Verification items for the finished model (mm, model axes). A direction names the side the tool comes from. Give positions to 0.01 mm unless a question says otherwise; leave off trailing zeros. Loops run counter-clockwise (first coordinate to the right, second up) from the corner with the lowest first, then second, coordinate; pieces in that order, holes last. Notation, with made-up numbers: (81, 89) - (87, 89) arc R35 ccw to (87, 122) - close; hole circle Ø4 at (-8, 12.25). An arc over 180 degrees is marked (long way). Use one line per item in the form item = value.
```python
from build123d import *

# Parameters (mm, degrees)
SKETCH1_W               = 58.8
SKETCH1_H               = 8
BOSS_EXTRUDE1_DEPTH     = 25
BOSS_EXTRUDE1_2_DEPTH   = 25
SKETCH1_3_W             = 58.8
SKETCH1_3_H             = 33.8
SKETCH1_3_W_2           = 58.5
SKETCH1_3_H_2           = 33.5
BOSS_EXTRUDE2_DEPTH     = 5
SKETCH2_R               = 1.375
CUT_EXTRUDE1_DEPTH      = 5
CUT_EXTRUDE2_DEPTH      = 74
CUT_EXTRUDE2_DEPTH_BACK = 20
SKETCH3_R               = 1.375
SKETCH4_W               = 15
SKETCH4_H               = 15
CUT_EXTRUDE3_DEPTH      = 75
SKETCH5_W               = 49.8
SKETCH5_H               = 25
BOSS_EXTRUDE3_DEPTH     = 8
SKETCH6_R               = 1.375
CUT_EXTRUDE4_DEPTH      = 16
BOSS_EXTRUDE4_START     = 5
SKETCH7_W               = 66.8
SKETCH7_H               = 49.8
SKETCH7_R               = 1.375
BOSS_EXTRUDE4_DEPTH     = 5
SKETCH8_W               = 126.8
SKETCH8_H               = 109.8
SKETCH8_W_2             = 66.8
SKETCH8_H_2             = 49.8
BOSS_EXTRUDE5_DEPTH     = 10
BOSS_EXTRUDE6_DEPTH     = 15
SKETCH11_R              = 1.375
CUT_EXTRUDE5_DEPTH      = 55
SKETCH12_R              = 1.625
CUT_EXTRUDE6_DEPTH      = 55
SKETCH13_R              = 3
CUT_EXTRUDE7_DEPTH      = 5
CUT_EXTRUDE8_START      = -5
SKETCH14_R              = 3
CUT_EXTRUDE8_DEPTH      = 5
SKETCH15_R              = 3
CUT_EXTRUDE9_DEPTH      = 7
SKETCH16_R              = 4
CUT_EXTRUDE10_DEPTH     = 5
SKETCH17_R              = 3
CUT_EXTRUDE11_DEPTH     = 5
BODY_MOVE_COPY1_ANGLE   = 120


with BuildPart() as part:
    # Sketch1 → Boss-Extrude1 (new body)
    with BuildSketch(Plane(origin=(0, 0, 0), x_dir=(1, 0, 0), z_dir=(0, 1, 0))):
        with Locations((0, 20.9)):
            Rectangle(SKETCH1_W, SKETCH1_H)
    extrude(amount=BOSS_EXTRUDE1_DEPTH)



with BuildPart() as body_2:
    # Sketch1 → Boss-Extrude1 2 (new body)
    with BuildSketch(Plane(origin=(0, 0, 0), x_dir=(1, 0, 0), z_dir=(0, 1, 0))):
        with Locations((0, -20.9)):
            Rectangle(SKETCH1_W, SKETCH1_H)
    extrude(amount=BOSS_EXTRUDE1_2_DEPTH)


with BuildPart() as part_1:
    add(part.part)

    add(body_2.part)  # Boss-Extrude2 merges body 2
    # Sketch1_3 → Boss-Extrude2 (add)
    # profile 1 of 2: a face of its own
    with BuildSketch(Plane(origin=(0, 0, 0), x_dir=(1, 0, 0), z_dir=(0, 1, 0))):
        Rectangle(SKETCH1_3_W, SKETCH1_3_H)
        Rectangle(SKETCH1_3_W_2, SKETCH1_3_H_2, mode=Mode.SUBTRACT)
    # profile 2 of 2: a face of its own
    with BuildSketch(Plane(origin=(0, 0, 0), x_dir=(1, 0, 0), z_dir=(0, 1, 0))):
        Rectangle(SKETCH1_3_W_2, SKETCH1_3_H_2)
    extrude(amount=BOSS_EXTRUDE2_DEPTH)

    # Sketch2 → Cut-Extrude1 (cut)
    with BuildSketch(Plane.XZ):
        with Locations(Location((-26.05, 13.5, 0), (0, 0, 270))):
            Circle(SKETCH2_R)
        with Locations(Location((-26.05, -13.5, 0), (0, 0, 270))):
            Circle(SKETCH2_R)
        with Locations(Location((25.95, -13.5, 0), (0, 0, 270))):
            Circle(SKETCH2_R)
        with Locations(Location((25.95, 13.5, 0), (0, 0, 270))):
            Circle(SKETCH2_R)
    extrude(amount=-CUT_EXTRUDE1_DEPTH, mode=Mode.SUBTRACT)

    # Sketch3 → Cut-Extrude2 (cut, two sides: drawn at the far end of the back side and taken through both)
    with BuildSketch(Plane(origin=(0, 0, 16.9), x_dir=(-1, 0, 0), z_dir=(0, 0, -1)).offset(-CUT_EXTRUDE2_DEPTH_BACK)):
        with Locations(Location((-22.45, 19, 0), (0, 0, 180))):
            Circle(SKETCH3_R)
        with Locations(Location((9.55, 19, 0), (0, 0, 180))):
            Circle(SKETCH3_R)
    extrude(amount=CUT_EXTRUDE2_DEPTH + CUT_EXTRUDE2_DEPTH_BACK, mode=Mode.SUBTRACT)

    # Sketch4 → Cut-Extrude3 (cut)
    with BuildSketch(Plane(origin=(0, 0, -24.9), x_dir=(-1, 0, 0), z_dir=(0, 0, -1))):
        with Locations((-1.9, 12.5)):
            Rectangle(SKETCH4_W, SKETCH4_H)
    extrude(amount=-CUT_EXTRUDE3_DEPTH, mode=Mode.SUBTRACT)

    # Sketch5 → Boss-Extrude3 (add)
    with BuildSketch(Plane(origin=(29.4, 0, 0), x_dir=(0, 0, -1), z_dir=(1, 0, 0))):
        with Locations((0, 12.5)):
            Rectangle(SKETCH5_W, SKETCH5_H)
    extrude(amount=BOSS_EXTRUDE3_DEPTH)

    # Sketch6 → Cut-Extrude4 (cut)
    with BuildSketch(Plane(origin=(37.4, 0, 0), x_dir=(0, 0, -1), z_dir=(1, 0, 0))):
        with Locations((-10, 19)):
            Circle(SKETCH6_R)
        with Locations((10, 19)):
            Circle(SKETCH6_R)
    extrude(amount=-CUT_EXTRUDE4_DEPTH, mode=Mode.SUBTRACT)

    # Sketch7 → Boss-Extrude4 (add)
    with BuildSketch(Plane.XZ.offset(BOSS_EXTRUDE4_START)):
        with Locations((4, 0)):
            Rectangle(SKETCH7_W, SKETCH7_H)
        with Locations(Location((-26.05, 13.5, 0), (0, 0, 270))):
            Circle(SKETCH7_R, mode=Mode.SUBTRACT)
        with Locations(Location((25.95, 13.5, 0), (0, 0, 270))):
            Circle(SKETCH7_R, mode=Mode.SUBTRACT)
        with Locations(Location((25.95, -13.5, 0), (0, 0, 270))):
            Circle(SKETCH7_R, mode=Mode.SUBTRACT)
        with Locations(Location((-26.05, -13.5, 0), (0, 0, 270))):
            Circle(SKETCH7_R, mode=Mode.SUBTRACT)
    extrude(amount=-BOSS_EXTRUDE4_DEPTH)

    # Sketch8 → Boss-Extrude5 (add)
    with BuildSketch(Plane.XZ.offset(5)):
        with Locations((4, 0)):
            Rectangle(SKETCH8_W, SKETCH8_H)
        with Locations((4, 0)):
            Rectangle(SKETCH8_W_2, SKETCH8_H_2, mode=Mode.SUBTRACT)
    extrude(amount=-BOSS_EXTRUDE5_DEPTH)

    # Sketch9 → Boss-Extrude6 (add)
    with BuildSketch(Plane(origin=(0, 25, 0), x_dir=(1, 0, 0), z_dir=(0, 1, 0))):
        Polygon((37.4, -24.9), (37.4, 24.9), (9.4, 24.9), (9.4, 16.9), (29.4, 16.9), (29.4, -16.9), (9.4, -16.9), (9.4, -24.9), align=None)
    extrude(amount=BOSS_EXTRUDE6_DEPTH)

    # Sketch11 → Cut-Extrude5 (cut)
    with BuildSketch(Plane.XY.offset(24.9)):
        with Locations((22.45, 35)):
            Circle(SKETCH11_R)
    extrude(amount=-CUT_EXTRUDE5_DEPTH, mode=Mode.SUBTRACT)

    # Sketch12 → Cut-Extrude6 (cut)
    with BuildSketch(Plane(origin=(0, 5, 0), x_dir=(1, 0, 0), z_dir=(0, 1, 0))):
        with Locations(Location((-44.4, 39.9, 0), (0, 0, 270))):
            Circle(SKETCH12_R)
        with Locations(Location((52.4, 39.9, 0), (0, 0, 270))):
            Circle(SKETCH12_R)
        with Locations(Location((52.4, -39.9, 0), (0, 0, 270))):
            Circle(SKETCH12_R)
        with Locations(Location((-44.4, -39.9, 0), (0, 0, 270))):
            Circle(SKETCH12_R)
    extrude(amount=-CUT_EXTRUDE6_DEPTH, mode=Mode.SUBTRACT)

    # Sketch13 → Cut-Extrude7 (cut)
    with BuildSketch(Plane.XY.offset(24.9)):
        with Locations((-9.55, 19)):
            Circle(SKETCH13_R)
        with Locations((22.45, 35)):
            Circle(SKETCH13_R)
        with Locations((22.45, 19)):
            Circle(SKETCH13_R)
    extrude(amount=-CUT_EXTRUDE7_DEPTH, mode=Mode.SUBTRACT)

    # Sketch14 → Cut-Extrude8 (cut)
    with BuildSketch(Plane(origin=(0, 0, -24.9), x_dir=(-1, 0, 0), z_dir=(0, 0, -1)).offset(CUT_EXTRUDE8_START)):
        with Locations(Location((-22.45, 35, 0), (0, 0, 180))):
            Circle(SKETCH14_R)
        with Locations(Location((-22.45, 19, 0), (0, 0, 180))):
            Circle(SKETCH14_R)
        with Locations(Location((9.55, 19, 0), (0, 0, 180))):
            Circle(SKETCH14_R)
    extrude(amount=CUT_EXTRUDE8_DEPTH, mode=Mode.SUBTRACT)

    # Sketch15 → Cut-Extrude9 (cut)
    with BuildSketch(Plane.XZ.offset(5)):
        with Locations(Location((-26.05, 13.5, 0), (0, 0, 270))):
            Circle(SKETCH15_R)
        with Locations(Location((25.95, 13.5, 0), (0, 0, 270))):
            Circle(SKETCH15_R)
        with Locations(Location((25.95, -13.5, 0), (0, 0, 270))):
            Circle(SKETCH15_R)
        with Locations(Location((-26.05, -13.5, 0), (0, 0, 270))):
            Circle(SKETCH15_R)
    extrude(amount=-CUT_EXTRUDE9_DEPTH, mode=Mode.SUBTRACT)

    # Sketch16 → Cut-Extrude10 (cut)
    with BuildSketch(Plane(origin=(0, 5, 0), x_dir=(1, 0, 0), z_dir=(0, 1, 0))):
        with Locations(Location((-44.4, 39.9, 0), (0, 0, 270))):
            Circle(SKETCH16_R)
        with Locations(Location((52.4, 39.9, 0), (0, 0, 270))):
            Circle(SKETCH16_R)
        with Locations(Location((52.4, -39.9, 0), (0, 0, 270))):
            Circle(SKETCH16_R)
        with Locations(Location((-44.4, -39.9, 0), (0, 0, 270))):
            Circle(SKETCH16_R)
    extrude(amount=-CUT_EXTRUDE10_DEPTH, mode=Mode.SUBTRACT)

    # Sketch17 → Cut-Extrude11 (cut)
    with BuildSketch(Plane(origin=(37.4, 0, 0), x_dir=(0, 0, -1), z_dir=(1, 0, 0))):
        with Locations((-10, 19)):
            Circle(SKETCH17_R)
        with Locations((10, 19)):
            Circle(SKETCH17_R)
    extrude(amount=-CUT_EXTRUDE11_DEPTH, mode=Mode.SUBTRACT)


with BuildPart() as part_2:
    # Body-Move_Copy1: moved
    add(part_1.part.moved(Location((0, 0, 0))).rotate(Axis((8.5, 13, -4.5), (0.5773502691896252, -0.5773502691896272, -0.5773502691896252)), BODY_MOVE_COPY1_ANGLE))


solid = part_2.part
```
1. Section check D-D, the plane x = 9. Record the cut outline in (y, z), then the cut area to 3 significant figures.
Result set:
outline = (-45.9, -22.5) - (80.9, -22.5) - (80.9, -12.5) - (-7.9, -12.5) - (-7.9, 22.5) - (-15.9, 22.5) - (-15.9, -12.5) - (-45.9, -12.5) - close
area = 1,550 mm²
2. Section check C-C, the plane y = 65.9. Record the cut outline in (x, z) (3 decimals).
Result set:
outline = (-50.9, -22.5) - (-37.525, -22.5) - (-37.525, -17.5) - (-39.9, -17.5) - (-39.9, -12.5) - (-50.9, -12.5) - close; (-34.275, -22.5) - (42.275, -22.5) - (42.275, -17.5) - (39.9, -17.5) - (39.9, -12.5) - (-31.9, -12.5) - (-31.9, -17.5) - (-34.275, -17.5) - close; (45.525, -22.5) - (58.9, -22.5) - (58.9, -12.5) - (47.9, -12.5) - (47.9, -17.5) - (45.525, -17.5) - close
3. Scan lines: probe 1 along X at (y, z) = (-4.45, -20); probe 2 along Y at (x, z) = (17.5, -18); probe 3 along X at (y, z) = (9.5, 11.5). Record each from-to range of solid material in increasing order.
Result set:
probe_1 = -50.9 to -12.5, -6.5 to 14.5, 20.5 to 58.9
probe_2 = -45.9 to -7.45, -1.45 to 44.55, 50.55 to 80.9
probe_3 = -20.9 to -12.9, 20.9 to 28.9
4. Depth check by flat-ended pin: pin 1 Ø9.5 at (y, z) = (-0.95, 17.5) entering from -X; pin 2 Ø5 at (x, y) = (43.9, -30.9) entering from +Z; pin 3 Ø9.5 at (y, z) = (31.05, 1.5) entering from +X. Enter the tip coordinate at first touch or a pass-through.
Result set:
pin_1 = -20.9
pin_2 = -17.5
pin_3 = 28.9
5. Tool access check on faces 4 (the flat face through (-17, 19, 2.5)), 5 (the cylindrical face through (-12.497, -4.582, -19.049)), 6 (the flat face through (23.9, 30, 3)), 7 (the flat face through (4, -15.9, 5)), 8 (the cylindrical face through (-18.435, -2.334, -1.162)). Record the directions out of +Z, -Z, +X, -X, +Y, -Y that give a thin tool (end or side, any length) a straight path to the whole face; none if there is none.
Result set:
face_4 = +X, -X
face_5 = -Z
face_6 = +X
face_7 = +Z, +X, -X, -Y
face_8 = -X
6. Draft check along Y on faces 1 (the flat face through (5, -45.9, -18)), 2 (the cylindrical face through (-8.76, 46.39, -14.02)), 3 (the flat face through (-17, 12.1, 15)). Enter one of: released by +Y, released by -Y, zero draft, split by the parting line, or undercut.
Result set:
face_1 = released by -Y
face_2 = undercut
face_3 = released by +Y
7. Section check A-A, the plane x = 43.9. Record the cut outline in (y, z) (3 decimals), then the cut area to 3 significant figures.
Result set:
outline = (-45.9, -22.5) - (-32.525, -22.5) - (-32.525, -17.5) - (-34.9, -17.5) - (-34.9, -12.5) - (-45.9, -12.5) - close; (-29.275, -22.5) - (64.275, -22.5) - (64.275, -17.5) - (61.9, -17.5) - (61.9, -12.5) - (-26.9, -12.5) - (-26.9, -17.5) - (-29.275, -17.5) - close; (67.525, -22.5) - (80.9, -22.5) - (80.9, -12.5) - (69.9, -12.5) - (69.9, -17.5) - (67.525, -17.5) - close
area = 1,160 mm²
8. Section check B-B, the plane z = -4. Record the cut outline in (x, y), then the cut area to 3 significant figures.
Result set:
outline = (-20.9, -15.9) - (28.9, -15.9) - (28.9, 12.1) - (20.9, 12.1) - (20.9, -7.9) - (-12.9, -7.9) - (-12.9, 12.1) - (-20.9, 12.1) - close; (-20.9, 27.1) - (-12.9, 27.1) - (-12.9, 50.9) - (-20.9, 50.9) - close; (20.9, 27.1) - (28.9, 27.1) - (28.9, 50.9) - (20.9, 50.9) - close
area = 1,100 mm²
